Geometry: see drawing. Coordinates: mm, zero at the bounding-box minimum. Give positions to 0.01 mm unless a question says otherwise; leave off trailing zeros. Write each loop counter-clockwise with the first axis right and the second up, starting at its lowest first coordinate (ties: lowest second). Pieces come first, ordered by that corner, then holes. Notation, with made-up numbers: M 29.5,51 L 72.5,51 A8 cw 72.5,58 Z; hole C -31.5,-21 d9. An arc over 180 degrees is marked long. Use a Markdown table: item, result. Add a question column.
1) Section B-B on y = 1.1. State how many separate pieces and enclosed holes the cut face has, then the cut area to 3 significant figures.
2) Line query: line 1 (X direction, y = 2.15, z = 166.5) (1 decimal); line 2 (Z direction, x = 121, y = 0.25); line 3 (Z direction, x = 96.5, y = 1.95) (1 decimal). Output: solid intervals per line, ascending.
3) Pin query (flat end, axial travel): pin 1 (4 mm diameter, centred on x = 48.5, z = 153, fed in from -Y); pin 2 (1.5 mm diameter, centred on x = 126.5, y = 1.5, fed in from +Z) (1 decimal). Return the tip coordinate at first contact, or that it passes through.
4) Section D-D on x = 57.5. Return the cut outline in (y, z).
5) Section A-A on z = 123.5. Return the cut outline in (x, y).
6) Section C-C on z = 81.5. Return the cut outline in (x, y).
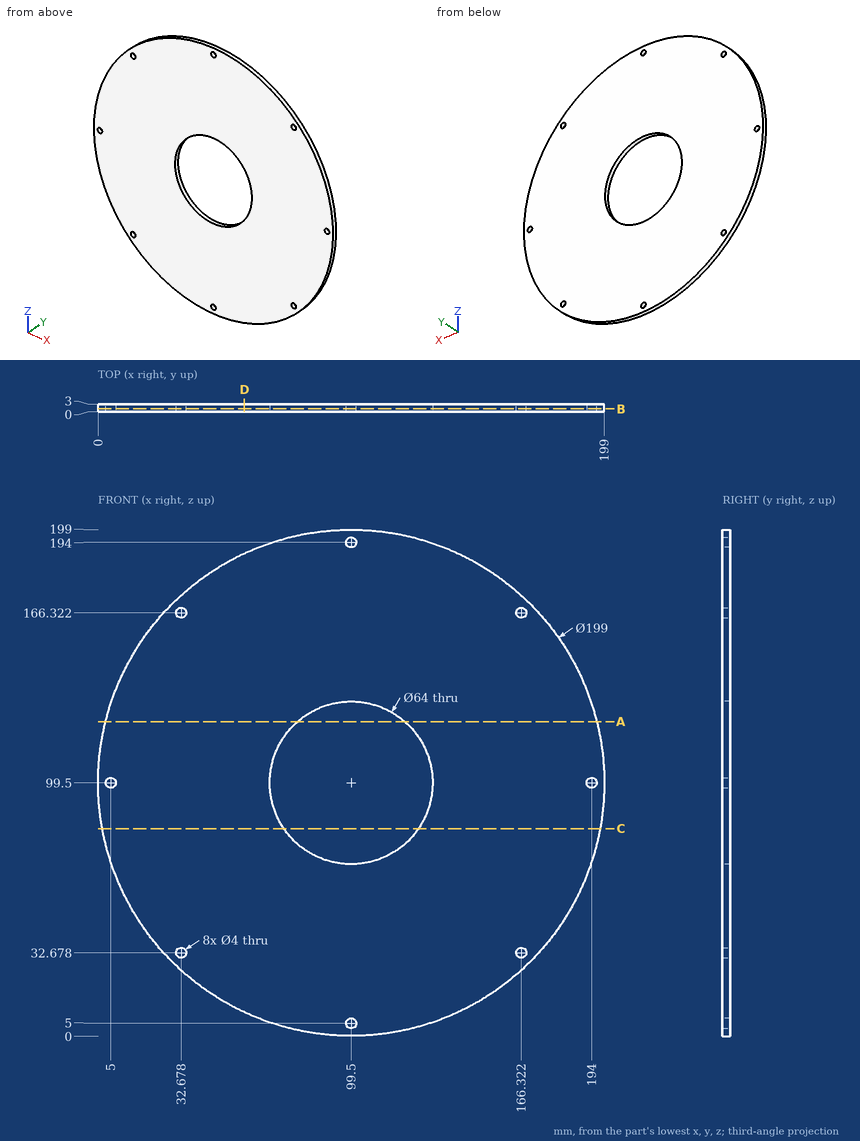
Found:
| question | item | result |
|---|---|---|
| 1 | separate pieces | 1 |
| 1 | enclosed holes | 9 |
| 1 | area | 27,800 mm² |
| 2 | line 1 | 25.9 to 30.7, 34.7 to 164.3, 168.3 to 173.1 |
| 2 | line 2 | 2.35 to 75.8, 123.2 to 196.65 |
| 2 | line 3 | 0 to 67.6, 131.4 to 199 |
| 3 | pin 1 | y = 0 |
| 3 | pin 2 | z = 195.5 |
| 4 | outline | M 0,9.3 L 3,9.3 L 3,189.7 L 0,189.7 Z |
| 5 | outline | M 2.94,0 L 78.33,0 L 78.33,3 L 2.94,3 Z; M 120.67,0 L 196.06,0 L 196.06,3 L 120.67,3 Z |
| 6 | outline | M 1.64,0 L 73.04,0 L 73.04,3 L 1.64,3 Z; M 125.96,0 L 197.36,0 L 197.36,3 L 125.96,3 Z |
